from build123d import *

# Parameters (mm, degrees)
F1_DEPTH    = 1.5
F3_DEPTH    = 3
F4_T1_DEPTH = 42.8345237792


# Not quite as in the source:
# - a fillet or chamfer that OpenCascade refuses, or shapes differently, is made with other operations: its cross-section is extruded or revolved along the edge and cut away or added


with BuildPart() as f1:
    # F0 (on Top) → F1 (new body, symmetric)
    with BuildSketch(Plane.XY):
        with BuildLine():
            Line((9.5752676601, 6.7411407109), (20.1104327648, 6.7411407109))
            ThreePointArc((20.1104327648, 6.7411407109), (-17.2170469432, 12.3873233035), (0, -21.2101976434))
            Line((0, -21.2101976434), (0, -11.7101976434))
            ThreePointArc((0, -11.7101976434), (10.3939602393, -5.3939150337), (9.5752676601, 6.7411407109))
        make_face()
        with BuildLine():
            Line((2, -3), (-2, -3))
            ThreePointArc((-2, -3), (-5, 0), (-2, 3))
            Line((-2, 3), (2, 3))
            ThreePointArc((2, 3), (5, 0), (2, -3))
        make_face(mode=Mode.SUBTRACT)
    extrude(amount=F1_DEPTH, both=True)

    # F2 (on face) → F3 (join)
    with BuildSketch(Plane.XY.offset(1.5)):
        with BuildLine():
            ThreePointArc((-19.9517186141, -7.19731953), (-21.2098366027, 0.1237552257), (-19.8663731217, 7.4296502651))
            Line((-19.8663731217, 7.4296502651), (-80.3057924461, 7.4296502651))
            Line((-80.3057924461, 7.4296502651), (-80.3057924461, -7.19731953))
            Line((-80.3057924461, -7.19731953), (-19.9517186141, -7.19731953))
        make_face()
    extrude(amount=-F3_DEPTH)

    # F4: fillet of radius 7.9669047558 on 2 edges, made by hand

    # F4_s2 → F4_t1 (cut)
    with BuildSketch(Plane.XY.offset(-21.4172618896)):
        with BuildLine():
            ThreePointArc((-72.3388876903, -7.19731953), (-77.9723400682, -4.863867152), (-80.3057924461, 0.7695852259))
            Line((-80.3057924461, 0.7695852259), (-80.3057924461, -7.19731953))
            Line((-80.3057924461, -7.19731953), (-72.3388876903, -7.19731953))
        make_face()
        with BuildLine():
            ThreePointArc((-72.3388876903, 7.4296502651), (-77.9723400682, 5.0961978872), (-80.3057924461, -0.5372544907))
            Line((-80.3057924461, -0.5372544907), (-80.3057924461, 7.4296502651))
            Line((-80.3057924461, 7.4296502651), (-72.3388876903, 7.4296502651))
        make_face()
    extrude(amount=F4_T1_DEPTH, mode=Mode.SUBTRACT)


solid = f1.part
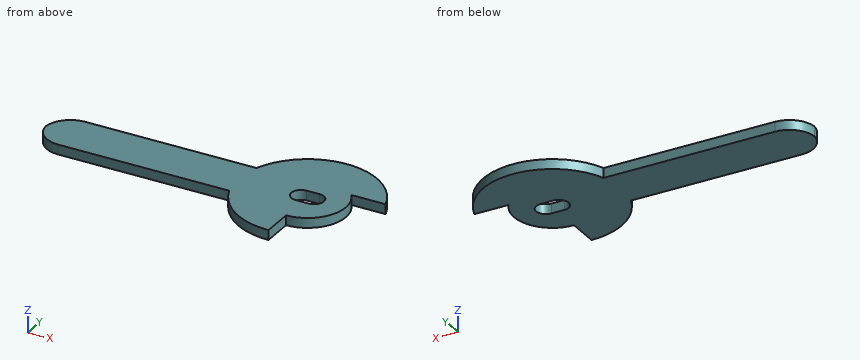
The listing builds one solid part. Answer for the finished solid, in the listing's coordinates (mm). Coordinates: 2 decimals unless noted, no trailing zeros. Order: outer loops, then holes, each group sorted by start corner. A loop starts at its lowest first (then second) coordinate and runs counter-clockwise, first axis right, second up.
Q1. Consider line 1 (X direction, y = 0, z = -0.7); line 2 (Y direction, x = -21.5, z = 1.3); line 3 (Y direction, x = -3, z = -0.3). Determine where each line is inside the solid, lowest interval first.
Q2. A cutting plane is placed at A-A, the plane z = 0.95. Write down the section's boundary in (x, y), and give its area (3 significant figures).
Q3. A cutting plane is placed at B-B, the plane y = 1.5. Write down the section's boundary in (x, z), and give its area (3 significant figures).
Q4. A cutting plane is placed at D-D, the plane y = -14. Write down the section's boundary in (x, z).
Q5. A cutting plane is placed at C-C, the plane x = -25. Write down the section's boundary in (y, z).
Q6. Given P1, Ø0.9, axis at x = -55.5, z = -0.5, coming from the -Y side; P2, Ø1, axis at y = 3, z = 1, coming from the +X side, each flat-ended and moving along its own axis, determine where each tip first touches the part or whether it passes through.
Answers follow:
1. line 1: x = -80.27 to -5, 5 to 11.71
1. line 2: y = -7.2 to 7.43
1. line 3: y = -21 to -2.83, 2.83 to 21
2. outline: (-80.28, 0.12) arc R7.97 ccw to (-72.34, -7.2) - (-19.95, -7.2) arc R21.21 ccw to (0, -21.21) - (0, -11.71) arc R11.71 ccw to (9.58, 6.74) - (20.11, 6.74) arc R21.21 ccw to (-19.87, 7.43) - (-72.34, 7.43) arc R7.97 ccw to start; hole (-2, -3) - (2, -3) arc R3 ccw to (2, 3) - (-2, 3) arc R3 ccw to start
2. area: 1,890 mm2
3. outline: (-80.04, -1.5) - (-4.6, -1.5) - (-4.6, 1.5) - (-80.04, 1.5) - close; (4.6, -1.5) - (11.61, -1.5) - (11.61, 1.5) - (4.6, 1.5) - close
3. area: 247 mm2
4. outline: (-15.93, -1.5) - (0, -1.5) - (0, 1.5) - (-15.93, 1.5) - close
5. outline: (-7.2, -1.5) - (7.43, -1.5) - (7.43, 1.5) - (-7.2, 1.5) - close
6. P1: stops at y = -7.2
6. P2: stops at x = 11.44
